Autodesk Inventor part; units mm, degrees
ref_plane "YZ Plane" through (0, 0, 0) normal (1, 0, 0) x (0, 1, 0)
ref_plane "XZ Plane" through (0, 0, 0) normal (0, 1, 0) x (-1, 0, 0)
ref_plane "XY Plane" through (0, 0, 0) normal (0, 0, 1) x (1, 0, 0)
sketch "Sketch1" plane through (0, 0, 0) normal (1, 0, 0) x (0, 1, 0)
  line L0 (4.5, -15.6) -> (4.5, 0)
  line L1 (4.5, 0) -> (-4.5, 0)
  line L2 (-4.5, 0) -> (-4.5, -15.6)
  line L3 (7.5, -15.6) -> (7.5, 3)
  line L4 (7.5, 3) -> (-7.5, 3)
  line L5 (-7.5, 3) -> (-7.5, -15.6)
  line L6 (-7.5, -15.6) -> (-4.5, -15.6)
  line L7 (4.5, -15.6) -> (7.5, -15.6)
  point P0 (0, 0)
  point P1 (0, 0)
  dimension "SliderWallWidth" = 3
  dimension "d18" = 9
  dimension "d19" = 15.6
extrude "Extrusion1" add sketch "Sketch1" along normal mid plane 120
sketch "Sketch2" plane through (-60, -7.5, -15.6) normal (0, -1, 0) x (1, 0, 0)
  line L0 (120, 18.6) -> (110, 18.6)
  line L1 (110, 18.6) -> (110, 15.6)
  line L2 (110, 15.6) -> (120, 15.6)
  line L3 (120, 15.6) -> (120, 18.6)
  dimension "ScrewPlateSize" = 10
  dimension "ScrewPlateHeight" = 3
extrude "Extrusion2" add sketch "Sketch2" along normal blind 10
sketch "Sketch5" plane through (60, -7.5, 0) normal (0, 0, -1) x (-1, 0, 0)
  line L0 (10, -10) -> (0, -10) construction
  line L1 (10, 0) -> (10, -10) construction
  circle A0 centre (5, -5) radius 2.5
  point P0 (60, 7.5)
  point P1 (10, -5)
  point P2 (5, -10)
  dimension "ScrewHoleDia" = 5
extrude "Extrusion4" cut sketch "Sketch5" against normal through all
chamfer "Chamfer2" distance 1.5 angle 45 1 edges at (57.5, -12.5, 0)
mirror "Mirror2" about plane through (0, 0, 0) normal (0, 1, 0) of "Extrusion4", "Chamfer2", "Extrusion2"
mirror "Mirror3" about plane through (0, 0, 0) normal (1, 0, 0) of "Extrusion4", "Chamfer2", "Extrusion2", "Mirror2"
equation "\"d18\" = RackWidth + 2 * RackOffset"
equation "\"d19\" = RackHeight"
equation "\"d3\" = RackLength"
equation "\"d9\" = ScrewPlateSize"
equation "\"RackOffset\" = 0.5"
properties part number "RackSlider"
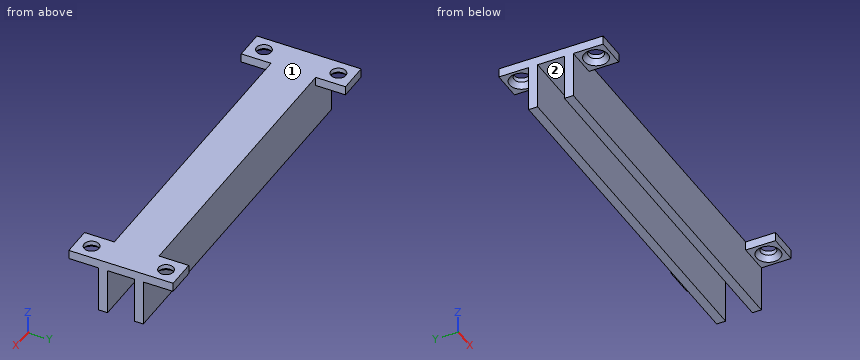
For this review, take the finished solid that the model builds, in its own axes (mm). Face numbers are marked on the shaded views. Round coordinates to 2 decimals unless told otherwise and drop trailing zeros. Loops run counter-clockwise (first coordinate to the right, second up) from the corner with the lowest first, then second, coordinate; pieces in that order, holes last. Notation, with made-up numbers: (58, -13) - (93, -13) arc R22 ccw to (93, 6) - close; hole circle Ø5 at (86.25, 85.25). An arc over 180 degrees is marked (long way). One line per question, with ' | ' between items.
Q1. Take a section at B-B (z = -3.5). Give the boundary of the cut face in (x, y).
Taken from the geometry:
outline: (-60, -7.5) - (60, -7.5) - (60, -4.5) - (-60, -4.5) - close; (-60, 4.5) - (60, 4.5) - (60, 7.5) - (-60, 7.5) - close
Q2. Take a section at C-C (x = 55). Give the boundary of the cut face in (y, z).
Taken from the geometry:
outline: (-17.5, 0) - (-16.5, 0) - (-15, 1.5) - (-15, 3) - (-17.5, 3) - close; (-10, 1.5) - (-8.5, 0) - (-7.5, 0) - (-7.5, -15.6) - (-4.5, -15.6) - (-4.5, 0) - (4.5, 0) - (4.5, -15.6) - (7.5, -15.6) - (7.5, 0) - (8.5, 0) - (10, 1.5) - (10, 3) - (-10, 3) - close; (15, 1.5) - (16.5, 0) - (17.5, 0) - (17.5, 3) - (15, 3) - close
Q3. Take a section at A-A (y = 12.5). Give the boundary of the cut face in (x, z), and give its area (3 significant figures).
Taken from the geometry:
outline: (-60, 0) - (-59, 0) - (-57.5, 1.5) - (-57.5, 3) - (-60, 3) - close; (-52.5, 1.5) - (-51, 0) - (-50, 0) - (-50, 3) - (-52.5, 3) - close; (50, 0) - (51, 0) - (52.5, 1.5) - (52.5, 3) - (50, 3) - close; (57.5, 1.5) - (59, 0) - (60, 0) - (60, 3) - (57.5, 3) - close | area: 25.5 mm²
Q4. For line 1 along Y through (x, z) = (55, 2.2); line 2 along X through (y, z) = (12.5, 1.95); line 3 along Y through (x, z) = (-20.5, -1.5), list the stretches that pass through material, from the lowest coordinate up. Write a range as [from, to].
Taken from the geometry:
line 1: y = [-17.5, -15], [-10, 10], [15, 17.5] | line 2: x = [-60, -57.5], [-52.5, -50], [50, 52.5], [57.5, 60] | line 3: y = [-7.5, -4.5], [4.5, 7.5]
Q5. Take a section at D-D (x = -32). Give the boundary of the cut face in (y, z).
Taken from the geometry:
outline: (-7.5, -15.6) - (-4.5, -15.6) - (-4.5, 0) - (4.5, 0) - (4.5, -15.6) - (7.5, -15.6) - (7.5, 3) - (-7.5, 3) - close
Q6. For pin 1 (9.5 mm diameter, centred on x = 16, z = -10.5, fed in from -Y); pin 2 (6 mm diameter, centred on x = 17, y = 13, fed in from -Z); pin 3 (6.5 mm diameter, centred on x = -55, y = -12.5, fed in from -Z); pin 4 (3 mm diameter, centred on x = -56.5, y = 13, fed in from -Z), all flat-tipped, find the tip position at first contact; note any pin that passes through.
Taken from the geometry:
pin 1: stops at y = -7.5 | pin 2: passes through | pin 3: stops at z = 0.75 | pin 4: stops at z = 0.92
Q7. The part is to be moulded in two halves that separate along Y. For the marked faces 1 and 2, say which applies: released by +Y, released by -Y, zero draft, split by the parting line, or undercut.
Taken from the geometry:
face 1: zero draft | face 2: undercut
